The listing builds one solid part. Answer for the finished solid, in the listing's coordinates (mm). Coordinates: 2 decimals unless noted, no trailing zeros. Loops run counter-clockwise (first coordinate to the right, second up) from the corner with the lowest first, then second, coordinate; pieces in that order, holes last. Notation, with made-up numbers: (56.5, 60) - (87.5, 60) arc R29 cw to (87.5, 87) - close; hole circle Ø9 at (-14.5, 52). An arc over 180 degrees is marked (long way). Return JSON: item names as keys, results as strings. Group by question number.
1. Section B-B (z = 24) is taken. Write down the section's boundary in (x, y), and give its area (3 significant figures).
2. Find the intervals of material crossed by line 1 along X through (y, z) = (54, 20.5); line 2 along Y through (x, z) = (30, 23); line 3 along X through (y, z) = (89, 28), in increasing order.
3. Section A-A (z = 12.5) is taken. Write down the section's boundary in (x, y).
4. Each of these flat-tipped pins is pushed along its axis until it touches: P1, Ø6, axis at x = 14, z = 30, coming from the +Y side; P2, Ø2, axis at x = -26.5, z = 17.5, coming from the -Y side; P3, Ø1.5, axis at x = -54, y = 129.5, coming from the +Z side. Where does it stop, or does it pass through?
```python
from build123d import *


with BuildPart() as f2:
    # F2: sweep along a path in F0
    with BuildLine(Plane.XY) as f2_path:
        ThreePointArc((0, 0), (-6.726505, 27.624275), (-25.4, 49.063656))
        ThreePointArc((-25.4, 49.063656), (-62.74699, 91.942418), (-76.2, 147.190969))
    # F1 (on Front) → F2 (sweep)
    with BuildSketch(Plane.XZ):
        Polygon((0, 0), (50.8, 0), (25.4, 43.994091), align=None)
    sweep(path=f2_path.line)


solid = f2.part
```
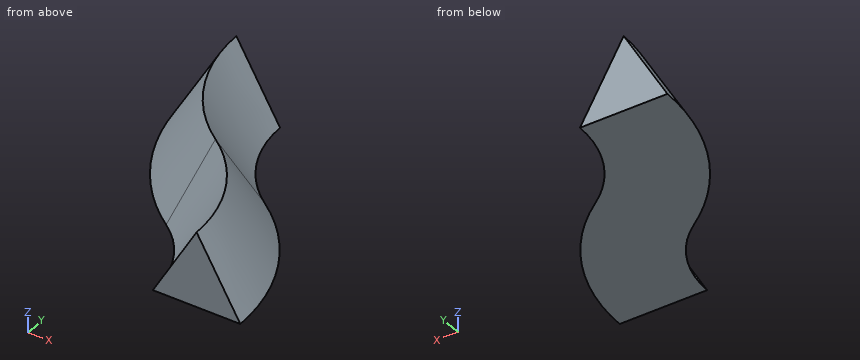
The answers:
{
 "1": {"outline": "(-62.34, 147.19) arc R106.32 ccw to (-17.4, 60.38) arc R73.94 cw to (13.86, 0) - (36.94, 0) arc R97.03 ccw to (-4.07, 79.23) arc R83.23 cw to (-39.26, 147.19) - close", "area": "3,980 mm2"},
 "2": {"line 1": "x = -12.58 to 22.95", "line 2": "y = 0 to 37.57", "line 3": "x = -42.23 to -18.72"},
 "3": {"outline": "(-68.98, 147.19) arc R112.96 ccw to (-21.23, 54.96) arc R67.3 cw to (7.22, 0) - (43.58, 0) arc R103.67 ccw to (-0.24, 84.65) arc R76.59 cw to (-32.62, 147.19) - close"},
 "4": {"P1": "stops at y = 61.74", "P2": "stops at y = 61.53", "P3": "stops at z = 37.01"}
}
